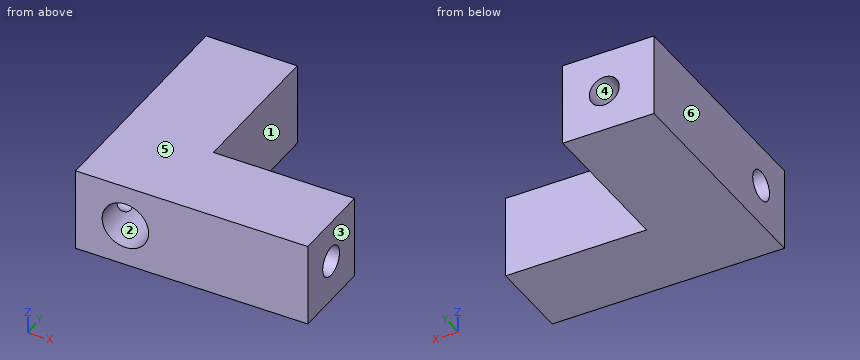
from build123d import *

# Parameters (mm, degrees)
F0_W     = 25
F0_H     = 25
F0_R     = 7
F0_R_2   = 4.5
F0_W_2   = 2.5
F1_DEPTH = 70
F2_DEPTH = 40
F0_W_3   = 42.5
F3_DEPTH = 25
F4_R     = 4.5
F5_DEPTH = 70.001


with BuildPart() as f1:
    # F0 (on Front) → F1 (new body)
    with BuildSketch(Plane.XZ):
        with Locations((-20, 0)):
            Rectangle(F0_W, F0_H)
        with Locations((-20, 0)):
            Circle(F0_R, mode=Mode.SUBTRACT)
        with Locations((-20, 0)):
            Circle(F0_R)
        with Locations((-20, 0)):
            Circle(F0_R_2, mode=Mode.SUBTRACT)
        with Locations((-33.75, 0)):
            Rectangle(F0_W_2, F0_H)
    extrude(amount=-F1_DEPTH)

    # F0 (on Front) → F2 (cut)
    with BuildSketch(Plane.XZ):
        with Locations((-20, 0)):
            Circle(F0_R)
        with Locations((-20, 0)):
            Circle(F0_R_2, mode=Mode.SUBTRACT)
    extrude(amount=-F2_DEPTH, mode=Mode.SUBTRACT)

    # F0 (on Front) → F3 (join)
    with BuildSketch(Plane.XZ):
        with Locations((13.75, 0)):
            Rectangle(F0_W_3, F0_H)
    extrude(amount=-F3_DEPTH)

    # F4 (on face) → F5 (cut, through all)
    with BuildSketch(Plane.YZ.offset(35)):
        with Locations((12.5, 0)):
            Circle(F4_R)
    extrude(amount=-F5_DEPTH, mode=Mode.SUBTRACT)


solid = f1.part
Build history of the part. All positions in model axes, mm. Face numbers are marked on the shaded views. A direction names the side the tool comes from. Coordinates: 2 decimals unless noted, no trailing zeros. Order: outer loops, then holes, each group sorted by start corner. A loop starts at its lowest first (then second) coordinate and runs counter-clockwise, first axis right, second up. Notation, with made-up numbers: (67, 37.5) - (110, 37.5) arc R14 ccw to (110, 48.5) - close; hole circle Ø10 at (-14.75, 67). An arc over 180 degrees is marked (long way). Write item = value, one per line. Start each with the question number.
1) Saw through at A-A on x = -20. Write the cut outline in (y, z).
2) Two-plate mould, pull along X, no slides. Class the marked faces 4, 5 and 6: pulls with the +X half, pulls with the -X half, needs draft (parallel to the pull), parting line crosses it, or undercut.
3) Saw through at B-B on y = 12.5. Write the cut outline in (x, z), then the cut area to 3 significant figures.
4) Saw through at C-C on z = 3. Write the cut outline in (x, y), then the cut area to 3 significant figures.
5) 3-axis set-ups, long thin cutter, end or side, ignore diameter. For the marked faces 1, 2 and 3: which of +Z, -Z, +X, -X, +Y, -Y reach the whole face in a straight line?
6) Wall check: line 1 along Z through (x, y) = (-20, 8); line 2 along Z through (x, y) = (-20, 58); line 3 along Y through (x, z) = (6, 0.25). Give the ranges that are in metal, low to high. Write a range as from..to.
7) Saw through at D-D on y = 64. Write the cut outline in (x, z), then the cut area to 3 significant figures.
8) Flat gauge pins, fed straight in: pin 1 Ø12 at (x, z) = (28, 8) entering from +Y; pin 2 Ø3 at (x, z) = (-12, -0.5) entering from -Y; pin 3 Ø12 at (y, z) = (44.5, 0.5) entering from +X. Where does each tip first touch, or does it go through?
From the geometry:
q1.outline = (0, -12.5) - (70, -12.5) - (70, -4.5) - (40, -4.5) - (40, -7) - (0, -7) - close; (0, 7) - (40, 7) - (40, 4.5) - (70, 4.5) - (70, 12.5) - (0, 12.5) - close
q2.face_4 = undercut
q2.face_5 = needs draft
q2.face_6 = pulls with the -X half
q3.outline = (-35, -12.5) - (35, -12.5) - (35, -4.5) - (-14.64, -4.5) arc R7 cw to (-25.36, -4.5) - (-35, -4.5) - close; (-35, 4.5) - (-25.36, 4.5) arc R7 cw to (-14.64, 4.5) - (35, 4.5) - (35, 12.5) - (-35, 12.5) - close
q3.area = 1,080 mm^2
q4.outline = (-35, 0) - (-26.32, 0) - (-26.32, 9.15) - (-35, 9.15) - close; (-35, 15.85) - (-26.32, 15.85) - (-26.32, 40) - (-23.35, 40) - (-23.35, 70) - (-35, 70) - close; (-16.65, 40) - (-13.68, 40) - (-13.68, 15.85) - (35, 15.85) - (35, 25) - (-7.5, 25) - (-7.5, 70) - (-16.65, 70) - close; (-13.68, 0) - (35, 0) - (35, 9.15) - (-13.68, 9.15) - close
q4.area = 1,900 mm^2
q5.face_1 = +Z, -Z, +X, +Y
q5.face_2 = -Y
q5.face_3 = +Z, -Z, +X, +Y, -Y
q6.line_1 = -12.5..-7, 7..12.5
q6.line_2 = -12.5..-4.5, 4.5..12.5
q6.line_3 = 0..8.01, 16.99..25
q7.outline = (-35, -12.5) - (-7.5, -12.5) - (-7.5, 12.5) - (-35, 12.5) - close; hole circle Ø9 at (-20, 0)
q7.area = 624 mm^2
q8.pin_1 = 25
q8.pin_2 = 0
q8.pin_3 = -7.5
